Here's the drawing with two shaded views (mm, measured from the low corner). I have some questions. A direction names the side the tool comes from. Coordinates: 2 decimals unless noted, no trailing zeros. Write each loop counter-clockwise with the first axis right and the second up, starting at its lowest first coordinate (ties: lowest second). Pieces come first, ordered by that corner, then holes. Notation, with made-up numbers: M 13.25,62.25 L 57.25,62.25 A26 ccw 57.25,97.25 Z; hole C 2.25,47 d9. An arc over 180 degrees is marked long. Use one line per item in the form item = value. Start each with the question number.
1. I want a section at B-B, the plane z = 36. List the corners of the cut face in (x, y) for me, plus the area to 3 significant figures.
2. Please list where these lines run through material, in increasing order: line 1 along X through (y, z) = (55, 30); line 2 along Z through (x, y) = (62.5, 42.5); line 3 along Z through (x, y) = (61, 4.5). Write a range as [from, to].
3. I want a section at A-A, the plane x = 14.5. List the corners of the cut face in (y, z) for me.
4. I want a section at D-D, the plane x = 86.5. List the corners of the cut face in (y, z) for me (1 decimal).
5. I want a section at C-C, the plane y = 63. List the corners of the cut face in (x, z) for me (1 decimal), plus the area to 3 significant figures.
6. I'm going to push flat-ended pins straight in: pin 1 Ø4 at (x, y) = (18.5, 27) entering from -Z; pin 2 Ø4 at (x, y) = (45.5, 38.5) entering from +Z; pin 3 Ø8 at (x, y) = (124.5, 43) entering from +Z (3 decimals); pin 4 Ø6.5 at (x, y) = (58.5, 30) entering from -Z. Where does each tip first touch, or does it pass through?
7. On a 3-axis mill with a long thin cutter (end or side, diameter ignored), from which of +Z, -Z, +X, -X, +Y, -Y can I reach the whole of each face in a straight line? I mean the marked faces 4, 5, 6, 7 and 8. Say none if no direction works.
8. Thinking about a two-plate mould opening in X: for the marked faces 1, 2 and 3, which applies, released by +X, released by -X, zero draft, split by the parting line, or undercut?
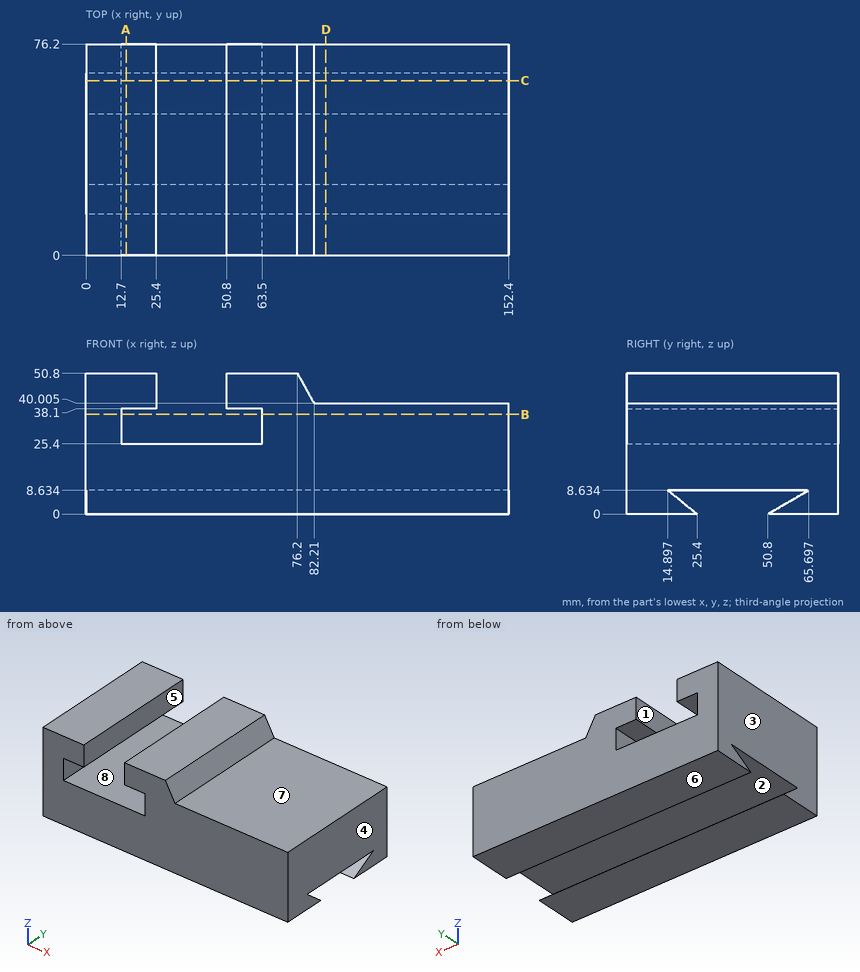
Answer list:
q1.outline = M 0,0 L 12.7,0 L 12.7,76.2 L 0,76.2 Z; M 63.5,0 L 152.4,0 L 152.4,76.2 L 63.5,76.2 Z
q1.area = 7,740 mm²
q2.line_1 = [0, 12.7], [63.5, 152.4]
q2.line_2 = [8.63, 25.4], [38.1, 50.8]
q2.line_3 = [0, 25.4], [38.1, 50.8]
q3.outline = M 0,0 L 25.4,0 L 14.9,8.63 L 65.7,8.63 L 50.8,0 L 76.2,0 L 76.2,25.4 L 0,25.4 Z; M 0,38.1 L 76.2,38.1 L 76.2,50.8 L 0,50.8 Z
q4.outline = M 0,0 L 25.4,0 L 14.9,8.6 L 65.7,8.6 L 50.8,0 L 76.2,0 L 76.2,40 L 0,40 Z
q5.outline = M 0,0 L 152.4,0 L 152.4,7.1 L 0,7.1 Z; M 0,8.6 L 152.4,8.6 L 152.4,40 L 82.2,40 L 76.2,50.8 L 50.8,50.8 L 50.8,38.1 L 63.5,38.1 L 63.5,25.4 L 12.7,25.4 L 12.7,38.1 L 25.4,38.1 L 25.4,50.8 L 0,50.8 Z
q5.area = 5,750 mm²
q6.pin_1 = 0
q6.pin_2 = 25.4
q6.pin_3 = 40.005
q6.pin_4 = 8.63
q7.face_4 = +Z, -Z, +X, +Y, -Y
q7.face_5 = +Z, +Y, -Y
q7.face_6 = -Z, +X, -X, +Y, -Y
q7.face_7 = +Z, +X, +Y, -Y
q7.face_8 = +Y, -Y
q8.face_1 = undercut
q8.face_2 = zero draft
q8.face_3 = released by -X
